CAD build for the part. Positions are in the model's coordinates, mm. A direction names the side the tool comes from. Coordinates: 2 decimals unless noted, no trailing zeros. Loops run counter-clockwise (first coordinate to the right, second up) from the corner with the lowest first, then second, coordinate; pieces in that order, holes last. Notation, with made-up numbers: (17.5, -24.5) -> (37.5, -24.5) arc R27 ccw to (37.5, 11.5) -> close; hole circle Ø5 at (64.5, 74.5). An arc over 180 degrees is marked (long way). Answer as a JSON object with one key per item and string values. Group by question number.
from build123d import *

# Parameters (mm, degrees)
F0_W      = 93.0914841592
F0_H      = 59.018785134
F1_DEPTH  = 25.4
F2_W      = 29.8136137426
F2_H      = 30.1178339869
F2_W_2    = 31.9431554526
F2_H_2    = 29.509392567
F3_DEPTH  = 25.4
F5_DEPTH  = 23.622
F6_W      = 28.9009511471
F6_H      = 55.4156415164
F7_DEPTH  = 25.4
F8_R      = 9.8202471376
F9_DEPTH  = 33.528
F10_R     = 8.1176194913
F10_R_2   = 8.5236088485
F11_DEPTH = 38.1
F12_R     = 8.0316605079
F13_DEPTH = 60.96


with BuildPart() as f1:
    # F0 (on Top) → F1 (new body)
    with BuildSketch(Plane.XY):
        with Locations((3.4985374659, -0.6084414199)):
            Rectangle(F0_W, F0_H)
    extrude(amount=F1_DEPTH)

    # F2 (on face) → F3 (cut)
    with BuildSketch(Plane.XY.offset(25.4)):
        with Locations((35.1374726743, -15.0589169934)):
            Rectangle(F2_W, F2_H)
        with Locations((-27.0756268874, -15.3631377034)):
            Rectangle(F2_W_2, F2_H_2)
    extrude(amount=-F3_DEPTH, mode=Mode.SUBTRACT)

    # F4 (on face) → F5 (join)
    with BuildSketch(Plane(origin=(-43.0472046137, 0, 0), x_dir=(0, -1, 0), z_dir=(-1, 0, 0))):
        Polygon((0, 0), (0.6084414199, 0), (0.6084414199, 55.2160292864), align=None)
        Polygon((0, 0), (0.6084414199, 55.2160292864), (-28.9009511471, 55.2160292864), (-28.9009511471, 0), align=None)
    extrude(amount=F5_DEPTH)

    # F6 (on face) → F7 (join)
    with BuildSketch(Plane.YZ.offset(50.0442795455)):
        with Locations((14.4504755735, 27.7078207582)):
            Rectangle(F6_W, F6_H)
    extrude(amount=F7_DEPTH)

    # F8 (on face) → F9 (cut)
    with BuildSketch(Plane.XY.offset(25.4)):
        with Locations((3.8986797445, -12.1688209474)):
            Circle(F8_R)
    extrude(amount=-F9_DEPTH, mode=Mode.SUBTRACT)

    # F10 (on Front) → F11 (cut)
    with BuildSketch(Plane.XZ):
        with Locations((-55.1201030612, 40.4613353312)):
            Circle(F10_R)
        with Locations((63.8301223516, 40.4613353312)):
            Circle(F10_R_2)
    extrude(amount=-F11_DEPTH, mode=Mode.SUBTRACT)

    # F12 (on Front) → F13 (cut)
    with BuildSketch(Plane.XZ):
        with Locations((-55.2160218358, 40.1571132243)):
            Circle(F12_R)
    extrude(amount=F13_DEPTH, mode=Mode.SUBTRACT)


solid = f1.part
Item 1: Pull direction Z, two halves, no side cores. Call faces 1 (the cylindrical face through (-61.56, 14.25, 35.52)), 2 (the flat face through (-55, 14, 55.216)), 3 (the cylindrical face through (67.763, 14.248, 32.899)), 4 (the flat face through (3, 12, 0)): +Z half, -Z half, draft (parallel to the pull), parting line (faces both ways), or undercut.
Item 2: Band-saw the part on C-C, the plane x = -52.5. List the corners of the cut face in (y, z).
Item 3: Band-saw the part on A-A, the plane z = 27.5. List the corners of the cut face in (x, y).
Item 4: Flat gauge pins, fed straight in: P1, Ø5, axis at x = 53, z = 48, coming from the -Y side; P2, Ø15.5, axis at x = 3.9, y = -12.17, coming from the +Z side; P3, Ø7.5, axis at y = -9.5, z = 18, coming from the +X side; P4, Ø17.5, axis at x = 1.5, y = -11, coming from the +Z side. Where does each tip first touch, or does it go through?
Item 5: 3-axis set-ups, long thin cutter, end or side, ignore diameter. For faces 5 (the flat face through (-45, -0.608, 21)), 6 (the flat face through (-43.047, 14, 41)), 7 (the cylindrical face through (-61.136, -0.3, 45.585)), 8 (the flat face through (54, 0, 21)): which of +Z, -Z, +X, -X, +Y, -Y reach the whole face in a straight line?
Item 6: Band-saw the part on B-B, the plane y = -13.5. List the corners of the cut face in (x, z).
Item 7: Drill centre lines: L1, parallel to X at y = 26, z = 29; L2, parallel to X at y = -26, z = 17; L3, parallel to Y at x = 60, z = 23. Where is each one in solid material? Low to high.
Item 8: Band-saw the part on D-D, the plane y = 22.5. List the corners of the cut face in (x, z), and give its area (3 significant figures).
Reply:
{
 "1": {"face 1": "undercut", "face 2": "+Z half", "face 3": "undercut", "face 4": "-Z half"},
 "2": {"outline": "(-0.61, 0) -> (28.9, 0) -> (28.9, 32.78) -> (0, 32.78) -> (0, 32.6) -> (-0.61, 32.6) -> close; (-0.61, 47.72) -> (0, 47.72) -> (0, 48.14) -> (28.9, 48.14) -> (28.9, 55.22) -> (-0.61, 55.22) -> close"},
 "3": {"outline": "(-66.67, -0.61) -> (-43.05, -0.61) -> (-43.05, 28.9) -> (-66.67, 28.9) -> close; (50.04, 0) -> (75.44, 0) -> (75.44, 28.9) -> (50.04, 28.9) -> close"},
 "4": {"P1": "y = 0", "P2": "through", "P3": "x = 20.23", "P4": "z = 25.4"},
 "5": {"face 5": "+Z, -Z, -X, -Y", "face 6": "+Z, +Y, -Y", "face 7": "-Y", "face 8": "+Z, -Z, +X, -Y"},
 "6": {"outline": "(-11.1, 0) -> (-5.83, 0) -> (-5.83, 25.4) -> (-11.1, 25.4) -> close; (13.63, 0) -> (20.23, 0) -> (20.23, 25.4) -> (13.63, 25.4) -> close"},
 "7": {"L1": "-66.67 to -43.05, 50.04 to 75.44", "L2": "-11.1 to 20.23", "L3": "0 to 28.9"},
 "8": {"outline": "(-66.67, 0) -> (75.44, 0) -> (75.44, 55.42) -> (50.04, 55.42) -> (50.04, 25.4) -> (-43.05, 25.4) -> (-43.05, 55.22) -> (-66.67, 55.22) -> close; hole circle Ø16.24 at (-55.12, 40.46); hole circle Ø17.05 at (63.83, 40.46)", "area": "4,640 mm²"}
}
